Source: CAD feature listing. Evaluate the final solid. Frame: model axes, mm. A direction names the side the tool comes from. Give positions to 0.01 mm unless a question says otherwise; leave off trailing zeros. Order: outer loops, then holes, each group sorted by start corner. A loop starts at its lowest first (then second) coordinate and runs counter-clockwise, first axis right, second up. Notation, with made-up numbers: (-1, 70.25) -> (36, 70.25) arc R16 ccw to (36, 77.25) -> close; hole circle Ø3 at (-26.5, 19). An arc over 180 degrees is marked (long way). Use one line per item in the form item = value. Start each with the question number.
Autodesk Inventor part; units mm, degrees
ref_plane "YZ Plane" through (0, 0, 0) normal (1, 0, 0) x (0, 1, 0)
ref_plane "XZ Plane" through (0, 0, 0) normal (0, 1, 0) x (-1, 0, 0)
ref_plane "XY Plane" through (0, 0, 0) normal (0, 0, 1) x (1, 0, 0)
sketch "Sketch1" plane through (0, 0, 0) normal (0, 0, 1) x (1, 0, 0)
  line L0 (0, 0) -> (-25, 0)
  line L1 (-25, 0) -> (-25, 4)
  line L2 (-25, 4) -> (-4, 4)
  line L3 (-4, 4) -> (-4, 23)
  line L4 (-4, 23) -> (0, 23)
  line L5 (0, 23) -> (0, 0)
  dimension "d0" = 25
  dimension "d1" = 4
  dimension "d2" = 23
extrude "Extrusion1" add sketch "Sketch1" along normal mid plane 240
sketch "Sketch2" plane through (-4, 4, 120) normal (-1, 0, 0) x (0, 0, 1)
  circle A0 centre (-225, 11) radius 3.5
  line L0 (-240, 0) -> (-240, 19)
  line L1 (-240, 19) -> (0, 19)
  circle A1 centre (-155, 11) radius 3.5
  circle A2 centre (-85, 11) radius 3.5
  circle A3 centre (-15, 11) radius 3.5
  line L2 (0, 19) -> (0, 0)
  point P0 (-120, -4)
  dimension "d5" = 7
  dimension "d6" = 15
  dimension "d7" = 8
  dimension "d8" = 15
  dimension "d9" = 70
  dimension "d10" = 70
extrude "Extrusion2" cut sketch "Sketch2" against normal blind 10
sketch "Sketch3" plane through (-25, 4, 120) normal (0, 1, 0) x (1, 0, 0)
  circle A0 centre (12.5, 7) radius 3.5
  line L0 (0, 240) -> (0, 0)
  line L1 (21, 0) -> (0, 0)
  circle A1 centre (12.5, 45) radius 3.5
  line L2 (16, 45) -> (16, 7)
  line L3 (9, 7) -> (9, 45)
  line L4 (21, 240) -> (21, 0) construction
  line L5 (21, 120) -> (0, 120) construction
  circle A2 centre (12.5, 233) radius 3.5
  circle A3 centre (12.5, 195) radius 3.5
  line L6 (16, 195) -> (16, 233)
  line L7 (9, 233) -> (9, 195)
  point P0 (25, 120)
  dimension "d13" = 7
  dimension "d14" = 12.5
  dimension "d15" = 7
  dimension "d16" = 38
extrude "Extrusion3" cut sketch "Sketch3" against normal blind 10
fillet "Fillet1" radius 5 1 edges at (0, 0, 0)
fillet "Fillet2" radius 10 4 edges at (-2, 23, -120) (-25, 2, -120) (-25, 2, 120) (-2, 23, 120)
sketch "Sketch4" plane through (-4, 4, 120) normal (0, 1, 0) x (1, 0, 0)
  line L0 (4, 120) -> (-21, 120) construction
  line L1 (-21, 230) -> (-21, 10) construction
  line L2 (0, 230) -> (0, 10)
  circle A0 centre (-7.65, 105.9) radius 7.65
  circle A1 centre (-7.65, 134.1) radius 7.65
  line L3 (-7.65, 141.75) -> (-7.65, 98.25) construction
  circle A2 centre (-7.65, 134.1) radius 5.4
  circle A3 centre (-7.65, 105.9) radius 5.4
  line L4 (4, 10) -> (4, 230) construction
  point P0 (-7.65, 120)
  point P1 (4, 120)
  dimension "d21" = 15.3
  dimension "d22" = 10.8
  dimension "d23" = 10.8
  dimension "d24" = 43.5
extrude "Extrusion4" add sketch "Sketch4" along normal blind 223
equation "\"d8\" = d6"
equation "\"d10\" = d9"
properties part number "beugel armsteun" material "Stainless Steel"
1) Pin query (flat end, axial travel): pin 1 (10 mm diameter, centred on x = -4.5, y = 116, fed in from +Z); pin 2 (12 mm diameter, centred on x = -10, y = 29.5, fed in from +Z); pin 3 (1.2 mm diameter, centred on y = 2.5, z = 92, fed in from +X). Return the tip coordinate at first contact, or that it passes through.
2) Material intervals for probe 1 along Z at (x, y) = (-11.65, 150.5); probe 2 along X at (y, z) = (132, -14); probe 3 along Z at (x, y) = (-7, 93.5), sorted ascending.
3) Cut plane D-D, the plane z = 2. Return the cut outline in (x, y).
4) Draft query along Z for faces 1 (the face through (-22.15, 2.03, 116.99)), 2 (the face through (-21.99, 2.03, -117.15)), 3 (the face through (-19.293, 113.939, -13.764)), 4 (the face through (-17, 227, -16)). Return one class per face: +Z half, -Z half, draft (parallel to the pull), parting line (faces both ways), or undercut.
5) Cut plane A-A, the plane z = -105. Return the cut outline in (x, y), plus the area to 3 significant figures.
6) Cut plane C-C, the plane z = 35. Return the cut outline in (x, y).
7) Cut plane B-B, the plane y = 167. Return the cut outline in (x, z).
8) Reachability of faces 5 (the face through (-2, 12.9, -37.8)), 6 (the face through (-17.045, 113.939, -13.863)) from +Z, -Z, +X, -X, +Y, -Y: full face, straight path, thin tool, end or side. Return the list, or none.
Output values:
q1.pin_1 = 21.44
q1.pin_2 = 21.75
q1.pin_3 = -0.38
q2.probe_1 = -21.75 to -19.5, -8.7 to -6.45, 6.45 to 8.7, 19.5 to 21.75
q2.probe_2 = -19.3 to -17.05, -6.25 to -4
q2.probe_3 = -20.17 to -16.85, -11.35 to -8.03, 8.03 to 11.35, 16.85 to 20.17
q3.outline = (-25, 0) -> (-5, 0) arc R5 ccw to (0, 5) -> (0, 23) -> (-4, 23) -> (-4, 4) -> (-25, 4) -> close
q4.face_1 = +Z half
q4.face_2 = -Z half
q4.face_3 = undercut
q4.face_4 = draft
q5.outline = (-25, 0) -> (-16, 0) -> (-16, 4) -> (-25, 4) -> close; (-9, 0) -> (-5, 0) arc R5 ccw to (0, 5) -> (0, 11.5) -> (-4, 11.5) -> (-4, 4) -> (-9, 4) -> close; (-4, 18.5) -> (0, 18.5) -> (0, 23) -> (-4, 23) -> close
q5.area = 115 mm^2
q6.outline = (-25, 0) -> (-5, 0) arc R5 ccw to (0, 5) -> (0, 11.5) -> (-4, 11.5) -> (-4, 4) -> (-25, 4) -> close; (-4, 18.5) -> (0, 18.5) -> (0, 23) -> (-4, 23) -> close
q7.outline = circle Ø15.3 at (-11.65, -14.1); circle Ø15.3 at (-11.65, 14.1); hole circle Ø10.8 at (-11.65, -14.1); hole circle Ø10.8 at (-11.65, 14.1)
q8.face_5 = +X, -X
q8.face_6 = +Y
